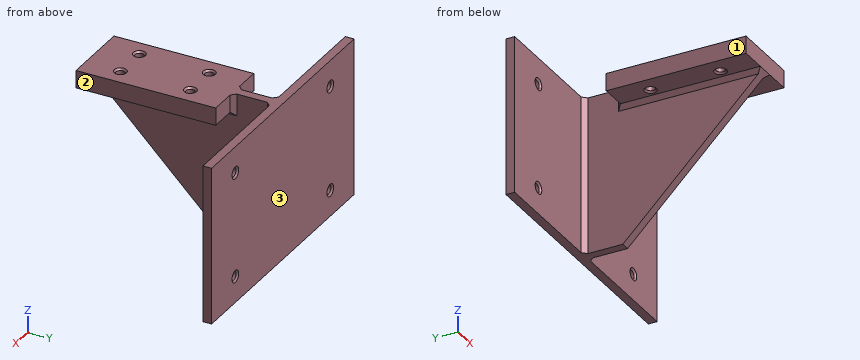
```python
from build123d import *

# Parameters (mm, degrees)
SKETCH1_W           = 40
SKETCH1_H           = 80
BOSS_EXTRUDE1_DEPTH = 10
SKETCH2_R           = 2.5
CUT_EXTRUDE1_DEPTH  = 10
BOSS_EXTRUDE2_DEPTH = 2.5
SKETCH4_W           = 150
SKETCH4_H           = 90
BOSS_EXTRUDE3_DEPTH = 2.5
CHAMFER1_SIZE       = 2.5
SKETCH5_R           = 2.5
CUT_EXTRUDE2_DEPTH  = 35
CHAMFER2_SIZE       = 1


with BuildPart() as part:
    # Sketch1 → Boss-Extrude1 (new body)
    with BuildSketch(Plane.XY):
        Rectangle(SKETCH1_W, SKETCH1_H)
    extrude(amount=BOSS_EXTRUDE1_DEPTH)

    # Sketch2 → Cut-Extrude1 (cut)
    with BuildSketch(Plane.XY.offset(10)):
        with Locations((-10, -20)):
            Circle(SKETCH2_R)
        with Locations(Location((10, -20, 0), (0, 0, 180))):
            Circle(SKETCH2_R)
        with Locations((10, 20)):
            Circle(SKETCH2_R)
        with Locations(Location((-10, 20, 0), (0, 0, 180))):
            Circle(SKETCH2_R)
    extrude(amount=-CUT_EXTRUDE1_DEPTH, mode=Mode.SUBTRACT)

    # Sketch3 → Boss-Extrude2 (add, symmetric)
    with BuildSketch(Plane(origin=(0, 0, 0), x_dir=(0, 0, -1), z_dir=(1, 0, 0))):
        Polygon((0, -40), (80, 40), (80, 65), (-10, 65), (-10, 40), (0, 40), align=None)
    extrude(amount=BOSS_EXTRUDE2_DEPTH, both=True)

    # Sketch4 → Boss-Extrude3 (add, symmetric)
    with BuildSketch(Plane(origin=(0, 65, 0), x_dir=(1, 0, 0), z_dir=(0, 1, 0))):
        with Locations((0, 35)):
            Rectangle(SKETCH4_W, SKETCH4_H)
    extrude(amount=BOSS_EXTRUDE3_DEPTH, both=True)

    # Chamfer1
    # the kernel refuses this chamfer: 2.5 mm, written as the material it adds along each edge
    with BuildSketch(Plane(origin=(-2.5, 40, 0), x_dir=(-0.9996219169112968, 0, 0.027495876610586372), z_dir=(0, -1, 0))) as chamfer1_piece_1_section:
        Polygon((CHAMFER1_SIZE * 0.999621916911, CHAMFER1_SIZE * 0.0274958766106), (-CHAMFER1_SIZE * 0.0274958766106, CHAMFER1_SIZE * 0.999621916911), (0, 0), align=None)
    chamfer1_piece_1 = extrude(amount=80, mode=Mode.PRIVATE)
    chamfer1_piece_1 = split(chamfer1_piece_1, bisect_by=Plane(origin=(-3.327144793, -19.384975846, -20.615024154), z_dir=(0, 0.7071067811865487, 0.7071067811865464)), keep=Keep.TOP, mode=Mode.PRIVATE)
    add(chamfer1_piece_1)
    with BuildSketch(Plane(origin=(-2.5, 40, 10), x_dir=(-0.9996219169112968, -0.0274958766105877, 0), z_dir=(0, 0, -1))) as chamfer1_piece_2:
        Polygon((CHAMFER1_SIZE * 0.999621916911, CHAMFER1_SIZE * 0.0274958766106), (-CHAMFER1_SIZE * 0.0274958766106, CHAMFER1_SIZE * 0.999621916911), (0, 0), align=None)
    extrude(amount=10)
    with BuildSketch(Plane(origin=(2.5, 40, 0), x_dir=(0.9996219169112968, 0, 0.027495876610586372), z_dir=(0, -1, 0))) as chamfer1_piece_3_section:
        Polygon((CHAMFER1_SIZE * 0.999621916911, -CHAMFER1_SIZE * 0.0274958766106), (-CHAMFER1_SIZE * 0.0274958766106, -CHAMFER1_SIZE * 0.999621916911), (0, 0), align=None)
    chamfer1_piece_3 = extrude(amount=80, mode=Mode.PRIVATE)
    chamfer1_piece_3 = split(chamfer1_piece_3, bisect_by=Plane(origin=(3.327144793, -19.384975846, -20.615024154), z_dir=(0, 0.7071067811865487, 0.7071067811865464)), keep=Keep.TOP, mode=Mode.PRIVATE)
    add(chamfer1_piece_3)
    with BuildSketch(Plane(origin=(2.5, 40, 10), x_dir=(0.9996219169112968, -0.0274958766105877, 0), z_dir=(0, 0, -1))) as chamfer1_piece_4:
        Polygon((CHAMFER1_SIZE * 0.999621916911, -CHAMFER1_SIZE * 0.0274958766106), (-CHAMFER1_SIZE * 0.0274958766106, -CHAMFER1_SIZE * 0.999621916911), (0, 0), align=None)
    extrude(amount=10)
    with BuildSketch(Plane(origin=(-2.5, 62.5, -80), x_dir=(0.027495876610586282, -0.9996219169112968, 0), z_dir=(0, 0, 1))) as chamfer1_piece_5:
        Polygon((CHAMFER1_SIZE * 0.999621916911, -CHAMFER1_SIZE * 0.0274958766106), (-CHAMFER1_SIZE * 0.0274958766106, -CHAMFER1_SIZE * 0.999621916911), (0, 0), align=None)
    extrude(amount=90)
    with BuildSketch(Plane(origin=(2.5, 62.5, -80), x_dir=(-0.027495876610586282, -0.9996219169112968, 0), z_dir=(0, 0, 1))) as chamfer1_piece_6:
        Polygon((CHAMFER1_SIZE * 0.999621916911, CHAMFER1_SIZE * 0.0274958766106), (-CHAMFER1_SIZE * 0.0274958766106, CHAMFER1_SIZE * 0.999621916911), (0, 0), align=None)
    extrude(amount=90)
    with BuildSketch(Plane(origin=(-2.5, 46.42920747, 0), x_dir=(-0.9996219169112968, 0, 0.027495876610586372), z_dir=(0, -1, 0))) as chamfer1_piece_7a_section:
        Polygon((CHAMFER1_SIZE * 0.999621916911, CHAMFER1_SIZE * 0.0274958766106), (-CHAMFER1_SIZE * 0.0274958766106, CHAMFER1_SIZE * 0.999621916911), (0, 0), align=None)
    chamfer1_piece_7a = extrude(amount=86.42920747, mode=Mode.PRIVATE)
    chamfer1_piece_7a = split(chamfer1_piece_7a, bisect_by=Plane(origin=(-3.324484067, 40, -0.824484067), z_dir=(0, 1, 0)), keep=Keep.TOP, mode=Mode.PRIVATE)
    with BuildSketch(Plane(origin=(-2.5, 40, 10), x_dir=(-0.9996219169112968, -0.0274958766105877, 0), z_dir=(0, 0, -1))) as chamfer1_piece_7b_section:
        Polygon((CHAMFER1_SIZE * 0.999621916911, CHAMFER1_SIZE * 0.0274958766106), (-CHAMFER1_SIZE * 0.0274958766106, CHAMFER1_SIZE * 0.999621916911), (0, 0), align=None)
    chamfer1_piece_7b = extrude(amount=16.42920747, mode=Mode.PRIVATE)
    chamfer1_piece_7b = split(chamfer1_piece_7b, bisect_by=Plane(origin=(-3.324484067, 40.824484067, 0), z_dir=(0, 0, -1)), keep=Keep.TOP, mode=Mode.PRIVATE)
    chamfer1_piece_7 = chamfer1_piece_7a & chamfer1_piece_7b
    add(chamfer1_piece_7)
    with BuildSketch(Plane(origin=(2.5, 46.42920747, 0), x_dir=(0.9996219169112968, 0, 0.027495876610586372), z_dir=(0, -1, 0))) as chamfer1_piece_8a_section:
        Polygon((CHAMFER1_SIZE * 0.999621916911, -CHAMFER1_SIZE * 0.0274958766106), (-CHAMFER1_SIZE * 0.0274958766106, -CHAMFER1_SIZE * 0.999621916911), (0, 0), align=None)
    chamfer1_piece_8a = extrude(amount=86.42920747, mode=Mode.PRIVATE)
    chamfer1_piece_8a = split(chamfer1_piece_8a, bisect_by=Plane(origin=(3.324484067, 40, -0.824484067), z_dir=(0, 1, 0)), keep=Keep.TOP, mode=Mode.PRIVATE)
    with BuildSketch(Plane(origin=(2.5, 40, 10), x_dir=(0.9996219169112968, -0.0274958766105877, 0), z_dir=(0, 0, -1))) as chamfer1_piece_8b_section:
        Polygon((CHAMFER1_SIZE * 0.999621916911, -CHAMFER1_SIZE * 0.0274958766106), (-CHAMFER1_SIZE * 0.0274958766106, -CHAMFER1_SIZE * 0.999621916911), (0, 0), align=None)
    chamfer1_piece_8b = extrude(amount=16.42920747, mode=Mode.PRIVATE)
    chamfer1_piece_8b = split(chamfer1_piece_8b, bisect_by=Plane(origin=(3.324484067, 40.824484067, 0), z_dir=(0, 0, -1)), keep=Keep.TOP, mode=Mode.PRIVATE)
    chamfer1_piece_8 = chamfer1_piece_8a & chamfer1_piece_8b
    add(chamfer1_piece_8)

    # Sketch5 → Cut-Extrude2 (cut, symmetric)
    with BuildSketch(Plane(origin=(0, 67.5, 0), x_dir=(1, 0, 0), z_dir=(0, 1, 0))):
        with Locations(Location((50, 65, 0), (0, 0, 90))):
            Circle(SKETCH5_R)
        with Locations(Location((50, 5, 0), (0, 0, 90))):
            Circle(SKETCH5_R)
        with Locations(Location((-50, 5, 0), (0, 0, 90))):
            Circle(SKETCH5_R)
        with Locations(Location((-50, 65, 0), (0, 0, 90))):
            Circle(SKETCH5_R)
    extrude(amount=CUT_EXTRUDE2_DEPTH, both=True, mode=Mode.SUBTRACT)

    # Chamfer2
    chamfer2_edges = [part.edges().sort_by_distance(p)[0] for p in [
        (-50, 62.5, -62.5),
        (-50, 67.5, -62.5),
        (-50, 62.5, -2.5),
        (-50, 67.5, -2.5),
        (50, 67.5, -2.5),
        (50, 62.5, -2.5),
        (50, 67.5, -62.5),
        (50, 62.5, -62.5),
        (-7.5, 20, 0),
        (-7.5, 20, 10),
        (7.5, 20, 0),
        (7.5, 20, 10),
        (12.5, -20, 0),
        (12.5, -20, 10),
        (-12.5, -20, 0),
        (-12.5, -20, 10),
    ]]
    chamfer(chamfer2_edges, length=CHAMFER2_SIZE)


solid = part.part
```
CAD build for the part. Positions are in the model's coordinates, mm. Face numbers are marked on the shaded views. A direction names the side the tool comes from. Coordinates: 2 decimals unless noted, no trailing zeros. Order: outer loops, then holes, each group sorted by start corner. A loop starts at its lowest first (then second) coordinate and runs counter-clockwise, first axis right, second up. Notation, with made-up numbers: (59, -6) - (90, -6) arc R21 ccw to (90, 8) - close; hole circle Ø11 at (8, 53). An arc over 180 degrees is marked (long way). Use a Markdown table: item, result. Add a question column.
(1) Which spindle directions (+Z, -Z, +X, -X, +Y, -Y) get a long thin tool onto all of the face, cutting with end or side? Do the marked faces 1, 2 and 3. Say none if no direction does.
(2) Flat gauge pins, fed straight in: pin 1 (5 mm diameter, centred on y = 10, z = 7, fed in from -X); pin 2 (3 mm diameter, centred on y = 18.5, z = 6, fed in from +X); pin 3 (21 mm diameter, centred on x = 38, z = -18, fed in from -Y); pin 4 (3 mm diameter, centred on x = -10, y = -20, fed in from +Z). Where does each tip first touch, or does it go through?
(3) Saw through at A-A (x = 50). Give the cut face in (y, z), then the cut area to 3 significant figures.
(4) Saw through at B-B (y = -20). Give the cut face in (x, z), then the cut area to 3 significant figures.
(5) Saw through at C-C (z = -65). Give the cut face in (x, y).
(6) Saw through at D-D (z = 3). Give the cut face in (x, y), then the cut area to 3 significant figures.
(7) Drill centre lines: line 1 along Z through (x, y) = (50, 64.5); line 2 along X through (y, z) = (64.85, -65); line 3 along Y through (x, z) = (10, 6). Where is each one in solid material? Low to high. Write a range as [from, to].
Solved:
| question | item | result |
|---|---|---|
| 1 | face 1 | +Z, -Z, -X, -Y |
| 1 | face 2 | +Z, -Z, +X, -Y |
| 1 | face 3 | +Z, -Z, +X, -X, +Y |
| 2 | pin 1 | stops at x = -20 |
| 2 | pin 2 | stops at x = 20 |
| 2 | pin 3 | stops at y = 62.5 |
| 2 | pin 4 | passes through |
| 3 | outline | (62.5, -80) - (67.5, -80) - (67.5, -68.5) - (66.5, -67.5) - (63.5, -67.5) - (62.5, -68.5) - close; (62.5, -61.5) - (63.5, -62.5) - (66.5, -62.5) - (67.5, -61.5) - (67.5, -8.5) - (66.5, -7.5) - (63.5, -7.5) - (62.5, -8.5) - close; (62.5, -1.5) - (63.5, -2.5) - (66.5, -2.5) - (67.5, -1.5) - (67.5, 10) - (62.5, 10) - close |
| 3 | area | 396 mm² |
| 4 | outline | (-20, 0) - (-13.5, 0) - (-12.5, 1) - (-12.5, 9) - (-13.5, 10) - (-20, 10) - close; (-7.5, 1) - (-6.5, 0) - (-5, 0) - (-2.5, -2.5) - (-2.5, -20) - (2.5, -20) - (2.5, -2.5) - (5, 0) - (6.5, 0) - (7.5, 1) - (7.5, 9) - (6.5, 10) - (-6.5, 10) - (-7.5, 9) - close; (12.5, 1) - (13.5, 0) - (20, 0) - (20, 10) - (13.5, 10) - (12.5, 9) - close |
| 4 | area | 402 mm² |
| 5 | outline | (-75, 62.5) - (-53.5, 62.5) - (-52.5, 63.5) - (-52.5, 66.5) - (-53.5, 67.5) - (-75, 67.5) - close; (-47.5, 63.5) - (-46.5, 62.5) - (-5, 62.5) - (-2.5, 60) - (-2.5, 25) - (2.5, 25) - (2.5, 60) - (5, 62.5) - (46.5, 62.5) - (47.5, 63.5) - (47.5, 66.5) - (46.5, 67.5) - (-46.5, 67.5) - (-47.5, 66.5) - close; (52.5, 63.5) - (53.5, 62.5) - (75, 62.5) - (75, 67.5) - (53.5, 67.5) - (52.5, 66.5) - close |
| 6 | outline | (-75, 62.5) - (-5, 62.5) - (-2.5, 60) - (-2.5, 42.5) - (-5, 40) - (-20, 40) - (-20, -40) - (20, -40) - (20, 40) - (5, 40) - (2.5, 42.5) - (2.5, 60) - (5, 62.5) - (75, 62.5) - (75, 67.5) - (-75, 67.5) - close; hole circle Ø5 at (-10, -20); hole circle Ø5 at (-10, 20); hole circle Ø5 at (10, -20); hole circle Ø5 at (10, 20) |
| 6 | area | 4,000 mm² |
| 7 | line 1 | z = [-80, -67.5], [-62.5, -7.5], [-2.5, 10] |
| 7 | line 2 | x = [-75, -52.5], [-47.5, 47.5], [52.5, 75] |
| 7 | line 3 | y = [-40, -22.5], [-17.5, 17.5], [22.5, 40], [62.5, 67.5] |
